Input: part model. Units: mm. Frame: model coordinates. Coordinates: 2 decimals unless noted, no trailing zeros. Order: outer loops, then holes, each group sorted by start corner. A loop starts at its lowest first (then second) coordinate and runs counter-clockwise, first axis right, second up. Notation, with made-up numbers: M 64.5,56 L 92.5,56 A27 ccw 92.5,75 Z; hole C 36,-16 d6. An arc over 180 degrees is marked long. One line per item, written item: value.
```python
from build123d import *

# Parameters (mm, degrees)
BOSS_EXTRUDE1_DEPTH        = 6
CUT_EXTRUDE1_DEPTH         = 7.0000001
M3_5_CLEARANCE_HOLE1_D     = 3.949564791
M3_5_CLEARANCE_HOLE1_DEPTH = 6.000055
FILLET1_R                  = 5.02065441
FILLET2_R                  = 74.958489821


with BuildPart() as part:
    # Sketch1 → Boss-Extrude1 (new body)
    with BuildSketch(Plane(origin=(0, 6, 0), x_dir=(1, 0, 0), z_dir=(0, 1, 0))):
        with BuildLine():
            Line((112.451900879, -119.772412512), (159.951903815, -37.500000848))
            add(Edge.make_bspline(
                [(159.951903815, -37.500000848), (162.089841538, -33.796778918), (165.842589826, -25.786061926), (169.244511458, -13.089917553), (169.999894602, -4.276058992), (169.999997188, -5.864e-06)],
                knots=[2.617993882, 2.617993882, 2.617993882, 2.617993882, 2.789036145, 2.970550387, 3.141592649, 3.141592649, 3.141592649, 3.141592649], degree=3))
            add(Edge.make_bspline(
                [(169.999997188, -5.864e-06), (169.999894602, 4.276047264), (169.244511458, 13.089905825), (165.842589826, 25.786050198), (162.089841538, 33.79676719), (159.951903815, 37.49998912)],
                knots=[3.141592658, 3.141592658, 3.141592658, 3.141592658, 3.31263492, 3.494149162, 3.665191425, 3.665191425, 3.665191425, 3.665191425], degree=3))
            Line((159.951903815, 37.49998912), (90.801278878, 157.272408343))
            Line((90.801278878, 157.272408343), (-90.8012615, 157.272408343))
            Line((-90.8012615, 157.272408343), (-159.951896595, 37.499994984))
            add(Edge.make_bspline(
                [(-159.951896595, 37.499994984), (-162.089834317, 33.796773054), (-165.842582605, 25.786056062), (-169.244504237, 13.08991169), (-169.999887381, 4.276053128), (-169.999989967, 0)],
                knots=[5.759586536, 5.759586536, 5.759586536, 5.759586536, 5.930628798, 6.11214304, 6.283185303, 6.283185303, 6.283185303, 6.283185303], degree=3))
            add(Edge.make_bspline(
                [(-169.999989967, 0), (-169.999887381, -4.276053128), (-169.244504237, -13.089911689), (-165.842582605, -25.786056062), (-162.089834317, -33.796773054), (-159.951896595, -37.499994984)],
                knots=[6.283185312, 6.283185312, 6.283185312, 6.283185312, 6.454227574, 6.635741816, 6.806784078, 6.806784078, 6.806784078, 6.806784078], degree=3))
            Line((-159.951896595, -37.499994984), (-112.451903815, -119.772412512))
            add(Edge.make_bspline(
                [(-112.451903815, -119.772412512), (-110.697042547, -122.811840435), (-108.72856528, -125.72791615), (-106.565705299, -128.491919084), (-106.17234227, -128.994613005), (-105.778979241, -129.497306926), (-105.385616213, -130.000000848)],
                knots=[0.523598778, 0.523598778, 0.523598778, 0.523598778, 0.663984963, 0.663984963, 0.663984963, 0.689517237, 0.689517237, 0.689517237, 0.689517237], degree=3))
            Line((-105.385616213, -130.000000848), (105.385613276, -130.000000848))
            add(Edge.make_bspline(
                [(105.385613276, -130.000000848), (105.778976305, -129.497306926), (106.172339333, -128.994613005), (106.565702362, -128.491919084), (108.728562343, -125.72791615), (110.69703961, -122.811840435), (112.451900879, -119.772412512)],
                knots=[2.452075416, 2.452075416, 2.452075416, 2.452075416, 2.477607691, 2.477607691, 2.477607691, 2.617993876, 2.617993876, 2.617993876, 2.617993876], degree=3))
        make_face()
    extrude(amount=-BOSS_EXTRUDE1_DEPTH)

    # Sketch2 → Cut-Extrude1 (cut, through all)
    with BuildSketch(Plane.XZ):
        Polygon((3.5, -157.27241336), (3.5, -140.27241336), (30, -140.27241336), (30, -126.27241336), (-30, -126.27241336), (-30, -140.27241336), (-3.5, -140.27241336), (-3.5, -157.27241336), align=None)
    extrude(amount=-CUT_EXTRUDE1_DEPTH, mode=Mode.SUBTRACT)

    # M3.5 Clearance Hole1
    with Locations(Plane(origin=(0, 0, 0), x_dir=(-1, 0, 0), z_dir=(0, -1, 0))):
        with Locations((98, -109.219962871), (-98, 102.438237129), (98, 102.438237129), (0, 102.438237129), (0, -109.219962871), (0, 3.7129e-05), (-97.9932, -3.7129e-05), (97.9932, -3.7129e-05), (111.4552, 69.849962871), (111.4552, -3.7129e-05), (-111.4552, 69.849962871), (-111.4552, -3.7129e-05), (-98, -109.219962871), (131.4, 50.300037129), (-131.4, 50.300037129), (131.4, -70.199962871), (-131.4, -70.199962871), (131.4, 63.000037129), (-131.4, 63.000037129), (131.4, -57.499962871), (-131.4, -57.499962871), (15, 148.600037129), (-15, 148.600037129), (150.47, 38.100037129), (150.47, -38.099962871), (-150.47, 38.100037129), (-150.47, -38.099962871)):
            Hole(M3_5_CLEARANCE_HOLE1_D / 2, depth=M3_5_CLEARANCE_HOLE1_DEPTH)

    # Fillet1
    fillet1_edges = [part.edges().sort_by_distance(p)[0] for p in [
        (-105.385616213, 3, 130.000000848),
        (3.5, 3, -140.27241336),
        (-3.5, 3, -157.272408343),
        (-30, 3, -126.27241336),
        (3.5, 3, -157.272408343),
        (-30, 3, -140.27241336),
        (-3.5, 3, -140.27241336),
        (30, 3, -140.27241336),
        (105.385613276, 3, 130.000000848),
        (30, 3, -126.27241336),
    ]]
    fillet(fillet1_edges, radius=FILLET1_R)

    # Fillet2
    fillet2_edges = [part.edges().sort_by_distance(p)[0] for p in [
        (90.801278878, 3, -157.272408343),
        (-90.8012615, 3, -157.272408343),
    ]]
    fillet(fillet2_edges, radius=FILLET2_R)


solid = part.part
```
(1) Ray query, line 1 (Z direction, x = 10, y = 3.5); line 2 (Z direction, x = 131.4, y = 1.4); line 3 (Z direction, x = -149.5, y = 4.75). Return the intervals inside material, ascending. Write a range as from..to.
Data:
line 1: z = -157.27..-140.27, -126.27..130
line 2: z = -86.95..-64.97, -61.03..-52.27, -48.33..55.53, 59.47..68.23, 72.17..86.95
line 3: z = -55.6..-39.82, -36.38..36.38, 39.82..55.6
(2) Cut plane B-B on z = -91. Output: boundary loops of the cut face in (x, y), plus the area to 3 significant figures.
Data:
outline: M -129.06,0 L 129.06,0 L 129.06,6 L -129.06,6 Z
area: 1,550 mm2
(3) Cut plane A-A on y = 3. Give the number of separate pieces and of enclosed holes in the cut face, plus the area to 3 significant figures.
Data:
separate pieces: 1
enclosed holes: 27
area: 77,800 mm2
(4) First-contact query: pin 1 (3.5 mm diameter, centred on x = 150.47, z = -38.1, fed in from -Y); pin 2 (1.5 mm diameter, centred on y = 1.5, z = -123.5, fed in from -X); pin 3 (2 mm diameter, centred on x = -126, y = 2, fed in from -Z); pin 4 (2 mm diameter, centred on x = -102, y = 2, fed in from -Z). Flat tips, straight axial feed; report the tip coordinate or a pass-through.
Data:
pin 1: passes through
pin 2: stops at x = -110.64
pin 3: stops at z = -98.04
pin 4: stops at z = -134.84
